The drawing under review shows one solid part. Ordinate dimensions are in mm from its lowest x, y, z. Round coordinates to 2 decimals unless told otherwise and drop trailing zeros. Write each loop counter-clockwise with the first axis right and the second up, starting at its lowest first coordinate (ties: lowest second). Pieces come first, ordered by that corner, then holes. Notation, with made-up numbers: M 1.25,34 L 52.25,34 A24 cw 52.25,58 Z; hole C 3.25,49.25 d10. An arc over 180 degrees is marked long. Write item = value, one per line. Start each with the question number.
Item 1: Take a section at B-B, the plane x = 7. Give the boundary of the cut face in (y, z), plus the area to 3 significant figures.
Item 2: Take a section at C-C, the plane y = 121. Give the boundary of the cut face in (x, z), plus the area to 3 significant figures.
Item 3: To check wall thickness, follow line 1 along Y through (x, z) = (11, 2.05); line 2 along X through (y, z) = (105, 1.65). State the ranges of each line that lie inside material, in increasing order.
Item 4: Take a section at A-A, the plane z = 1.5. Give the boundary of the cut face in (x, y), plus the area to 3 significant figures.
Item 5: For pin 1 Ø0.9 at (y, z) = (128, 1) entering from +X; pin 2 Ø1.5 at (x, z) = (64, 2) entering from -Y; pin 3 Ø1.5 at (x, z) = (1.5, 1) entering from +Y, all flat-tipped, find the tip position at first contact; note any pin that passes through.
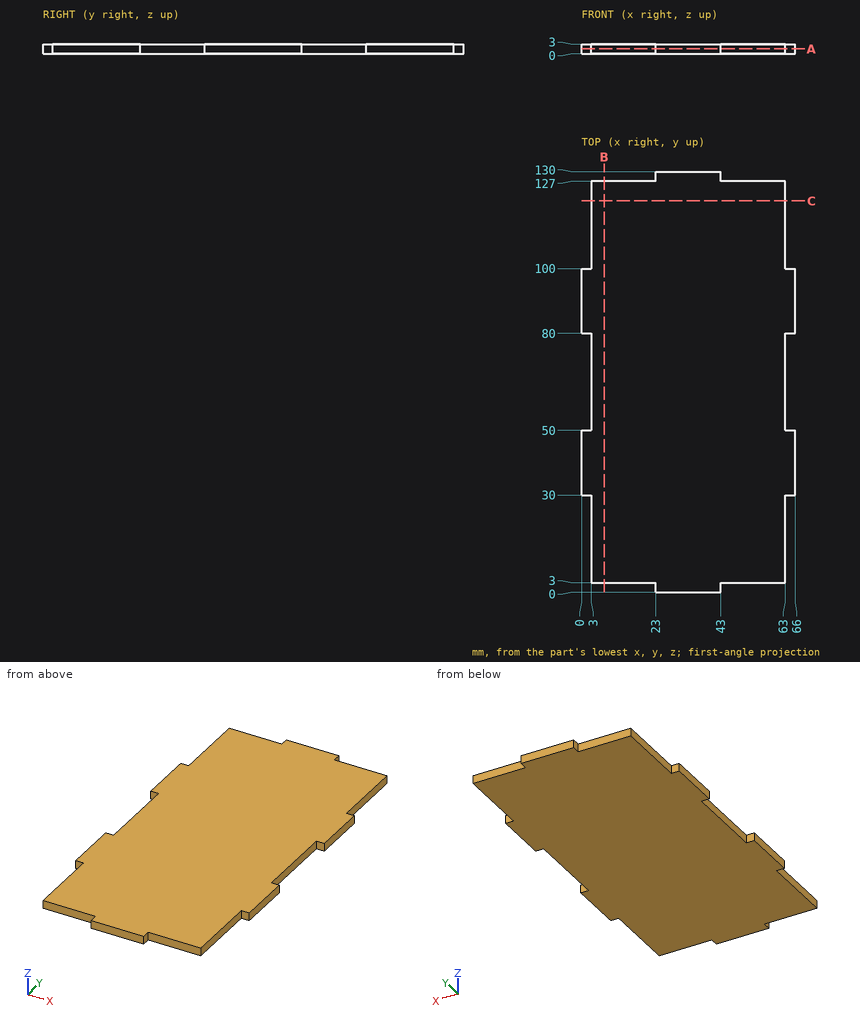
Response values:
q1.outline = M 3,0 L 127,0 L 127,3 L 3,3 Z
q1.area = 372 mm2
q2.outline = M 3,0 L 63,0 L 63,3 L 3,3 Z
q2.area = 180 mm2
q3.line_1 = 3 to 127
q3.line_2 = 3 to 63
q4.outline = M 0,30 L 3,30 L 3,3 L 23,3 L 23,0 L 43,0 L 43,3 L 63,3 L 63,30 L 66,30 L 66,50 L 63,50 L 63,80 L 66,80 L 66,100 L 63,100 L 63,127 L 43,127 L 43,130 L 23,130 L 23,127 L 3,127 L 3,100 L 0,100 L 0,80 L 3,80 L 3,50 L 0,50 Z
q4.area = 7,800 mm2
q5.pin_1 = 43
q5.pin_2 = 30
q5.pin_3 = 100
